from build123d import *

# Parameters (mm, degrees)
F3_START = -10
F2_R     = 3
F3_DEPTH = 20


with BuildPart() as f1:
    # F0 (on Front) → F1 (revolve)
    with BuildSketch(Plane.XZ):
        with BuildLine():
            Line((62.1, 0), (47.35, 0))
            Line((47.35, 0), (47.35, 3.5))
            Line((47.35, 3.5), (44.85, 3.5))
            Line((44.85, 3.5), (44.85, 31.2))
            Line((44.85, 31.2), (43.85, 31.2))
            Line((43.85, 31.2), (37.8303318608, 71.0116326655))
            ThreePointArc((37.8303318608, 71.0116326655), (36.1, 72.5), (34.3696681392, 71.0116326655))
            Line((34.3696681392, 71.0116326655), (27, 0))
            Line((27, 0), (35.3775171312, -61.4864782954))
            ThreePointArc((35.3775171312, -61.4864782954), (37.1394995022, -63), (38.8521475937, -61.4308708337))
            Line((38.8521475937, -61.4308708337), (43.1, -20.5))
            Line((43.1, -20.5), (58.7000275247, -19))
            ThreePointArc((58.7000275247, -19), (59.9249879423, -18.4212207992), (60.5, -17.194487527))
            Line((60.5, -17.194487527), (62.1, 0))
        make_face()
    revolve(axis=Axis((0, 0, -1.9075102699), (0, 0, -1)))

    # F2 (on Top) → F3 (cut)
    with BuildSketch(Plane.XY.offset(F3_START)):
        with Locations((0, 55)):
            Circle(F2_R)
        with Locations((-55, 0)):
            Circle(F2_R)
        with Locations((55, 0)):
            Circle(F2_R)
        with Locations((0, -55)):
            Circle(F2_R)
    extrude(amount=-F3_DEPTH, mode=Mode.SUBTRACT)


solid = f1.part
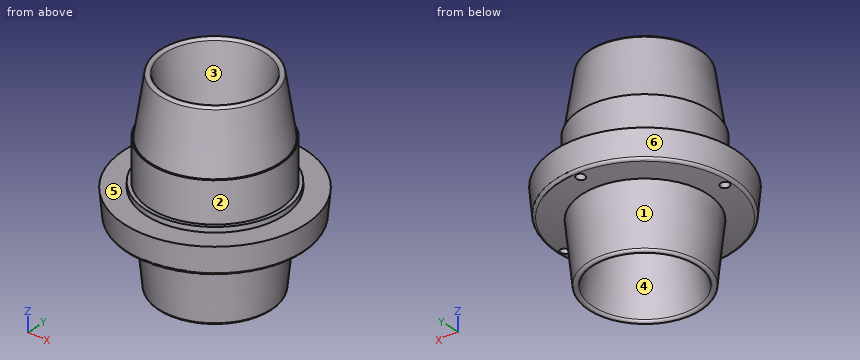
Can you work these out from the model? Positions are in its coordinate system, mm. Face numbers are marked on the shaded views. A direction names the side the tool comes from. Round coordinates to 2 decimals unless told otherwise and drop trailing zeros. Write each loop counter-clockwise with the first axis right and the second up, starting at its lowest first coordinate (ties: lowest second). Pieces come first, ordered by that corner, then holes. Notation, with made-up numbers: (56.25, 7.25) - (77.25, 7.25) arc R32 cw to (77.25, 46.25) - close; hole circle Ø8 at (21, 72.5). An arc over 180 degrees is marked (long way). Write each question's results on one line, items separated by ' | '. Start each with the question number.
1) For pin 1 Ø3.5 at (x, y) = (0, 55) entering from -Z; pin 2 Ø12 at (y, z) = (46.5, -19.5) entering from +X; pin 3 Ø10 at (y, z) = (-21.5, -43.5) entering from +X, each with a flat end and sliding along its axis, tell me the tip position at first contact or that it passes through.
2) Suppose I cut it at B-B (z = -6.5). List the corners of the cut face in (x, y) for me.
3) Suppose I cut it at A-A (z = 7.5). List the corners of the cut face in (x, y) for me.
4) We'd pull the mould along X, two halves only. Please class the marked faces 3, 4, 5 and 6: released by +X, released by -X, zero draft, split by the parting line, or undercut.
5) Which directions (+Z, -Z, +X, -X, +Y, -Y) give clear straight access to the entire face, cutting with the end or side of a thin tool? Please do the marked faces 1 and 2.
6) Please list where these lines run through material, in increasing order: line 1 (X direction, y = 0, z = -17.25); line 2 (Y direction, x = 0, z = -15.25); line 3 (Y direction, x = 0, z = -12.5).
Here are the results:
1) pin 1: stops at z = -10 | pin 2: stops at x = 44.56 | pin 3: stops at x = 37.29
2) outline: circle Ø122.99 at (0, 0); hole circle Ø55.77 at (0, 0)
3) outline: circle Ø89.7 at (0, 0); hole circle Ø55.56 at (0, 0)
4) face 3: undercut | face 4: undercut | face 5: zero draft | face 6: split by the parting line
5) face 1: -Z | face 2: +Z
6) line 1: x = -60.49 to -58, -52 to -29.35, 29.35 to 52, 58 to 60.49 | line 2: y = -60.68 to -58, -52 to -29.08, 29.08 to 52, 58 to 60.68 | line 3: y = -60.94 to -58, -52 to -28.7, 28.7 to 52, 58 to 60.94
